Can you work these out from the model? Positions are in its coordinate system, mm. A direction names the side the tool comes from. Give positions to 0.01 mm unless a question says otherwise; leave off trailing zeros. Loops run counter-clockwise (first coordinate to the right, second up) from the corner with the lowest first, then second, coordinate; pieces in that order, holes last. Notation, with made-up numbers: M 18,-9.5 L 73,-9.5 A19 ccw 73,-3.5 Z; hole C 54,-40 d9. An arc over 180 degrees is marked long. Answer as a JSON object with one key per item and string values.
```python
from build123d import *

# Parameters (mm, degrees)
F2_DEPTH  = 0.15
F0_W      = 4
F0_H      = 0.8
F0_W_2    = 7
F0_H_2    = 6
F2_FACE_W = 4
F2_FACE_H = 0.8
F1_W      = 17
F1_H      = 16
F3_DEPTH  = 0.5


with BuildPart() as f2:
    # F0 (on Top) → F2 (new body)
    with BuildSketch(Plane.XY):
        Polygon((0.9, -0.5), (0.5, -3), (0.9, -5.5), (6.1, -5.5), (6.5, -3), (6.1, -0.5), align=None)
        Polygon((1.2410876448, -5.1), (0.9050876448, -3), (1.2410876448, -0.9), (5.7589123552, -0.9), (6.0949123552, -3), (5.7589123552, -5.1), align=None, mode=Mode.SUBTRACT)
    extrude(amount=F2_DEPTH)



with BuildPart() as f2b:
    # F0 (on Top) → F2, piece 2 (new body)
    with BuildSketch(Plane.XY):
        with Locations((3.5949123552, -3)):
            Rectangle(F0_W, F0_H)
    extrude(amount=F2_DEPTH)


with BuildPart() as f2_1:
    add(f2.part)

    add(f2b.part)  # F3 merges F2b
    # F0 (on Top) + F2_face (on face) + F1 (on Top) → F3 (join)
    with BuildSketch(Plane.XY):
        with Locations((3.5, -3)):
            Rectangle(F0_W_2, F0_H_2)
        Polygon((0.9, -5.5), (0.5, -3), (0.9, -0.5), (6.1, -0.5), (6.5, -3), (6.1, -5.5), align=None, mode=Mode.SUBTRACT)
        Polygon((0.9, -0.5), (0.5, -3), (0.9, -5.5), (6.1, -5.5), (6.5, -3), (6.1, -0.5), align=None)
        Polygon((1.2410876448, -5.1), (0.9050876448, -3), (1.2410876448, -0.9), (5.7589123552, -0.9), (6.0949123552, -3), (5.7589123552, -5.1), align=None, mode=Mode.SUBTRACT)
        Polygon((1.2410876448, -0.9), (0.9050876448, -3), (1.2410876448, -5.1), (5.7589123552, -5.1), (6.0949123552, -3), (5.7589123552, -0.9), align=None)
        with Locations((3.5949123552, -3)):
            Rectangle(F0_W, F0_H, mode=Mode.SUBTRACT)
        with Locations((3.5949123552, -3)):
            Rectangle(F0_W, F0_H)
    with BuildSketch(Plane(origin=(3.5949123552, -3, 0), x_dir=(1, 0, 0), z_dir=(0, 0, -1))):
        Rectangle(F2_FACE_W, F2_FACE_H)
    with BuildSketch(Plane.XY):
        with Locations((3.5, -3)):
            Rectangle(F1_W, F1_H)
    extrude(amount=-F3_DEPTH, dir=(0, 0, 1))


solid = f2_1.part
```
1) Suppose I cut it at D-D, the plane y = 1. Write out the boundary of the cut face in (x, z).
Answer list:
{"outline": "M -5,-0.5 L 12,-0.5 L 12,0 L -5,0 Z"}
2) Suppose I cut it at A-A, the plane x = 4. Write out the boundary of the cut face in (y, z).
Answer list:
{"outline": "M -11,-0.5 L 5,-0.5 L 5,0 L -0.5,0 L -0.5,0.15 L -0.9,0.15 L -0.9,0 L -2.6,0 L -2.6,0.15 L -3.4,0.15 L -3.4,0 L -5.1,0 L -5.1,0.15 L -5.5,0.15 L -5.5,0 L -11,0 Z"}
3) Please list where this line runs through material, in increasing order: line 1 along Z through (x, y) = (-3.5, -1.25). Write a range as from..to.
Answer list:
{"line 1": "-0.5..0"}
4) Suppose I cut it at C-C, the plane x = 9.5. Write out the boundary of the cut face in (y, z), and give its area (3 significant figures).
Answer list:
{"outline": "M -11,-0.5 L 5,-0.5 L 5,0 L -11,0 Z", "area": "8.00 mm^2"}
5) Suppose I cut it at B-B, the plane y = -1.5. Write out the boundary of the cut face in (x, z).
Answer list:
{"outline": "M -5,-0.5 L 12,-0.5 L 12,0 L 6.26,0 L 6.26,0.15 L 5.85,0.15 L 5.85,0 L 1.15,0 L 1.15,0.15 L 0.74,0.15 L 0.74,0 L -5,0 Z"}
6) Will this pin go through, and if not, where does the flat tip stop? pin 1 Ø8 at (x, y) = (-3, 2.5) entering from +Z.
Answer list:
{"pin 1": "z = 0"}
7) For faces 1 (the flat face through (3, -3, -0.5)), 2 (the flat face through (3, 1, 0)), which set-ups out of +Z, -Z, +X, -X, +Y, -Y let a thin tool reach every point of the face, with its end or its side?
Answer list:
{"face 1": "-Z, +X, -X, +Y, -Y", "face 2": "+Z"}
